Geometry check sheet. Reference: the model listing, model coordinates, mm. A direction names the side the tool comes from. Coordinates: 2 decimals unless noted, no trailing zeros. Loops run counter-clockwise (first coordinate to the right, second up) from the corner with the lowest first, then second, coordinate; pieces in that order, holes last. Notation, with made-up numbers: M 31,37 L 86,37 A13 cw 86,42 Z; hole C 44,42.5 d5. An arc over 180 degrees is marked long. Use CSV: the item, a comma, the result in double quotes.
```python
from build123d import *

# Parameters (mm, degrees)
F0_W     = 457.2
F0_H     = 139.7
F1_DEPTH = 19.05
F2_W     = 19.05
F2_H     = 12.7
F3_DEPTH = 139.701
F4_W     = 19.05
F4_H     = 12.7
F5_DEPTH = 139.701


with BuildPart() as f1:
    # F0 (on Front) → F1 (new body)
    with BuildSketch(Plane.XZ):
        with Locations((-228.6, 69.85)):
            Rectangle(F0_W, F0_H)
    extrude(amount=F1_DEPTH)

    # F2 (on face) → F3 (cut, through all)
    with BuildSketch(Plane.XY.offset(139.7)):
        with Locations((-9.525, -6.35)):
            Rectangle(F2_W, F2_H)
    extrude(amount=-F3_DEPTH, mode=Mode.SUBTRACT)

    # F4 (on face) → F5 (cut, through all)
    with BuildSketch(Plane.XY.offset(139.7)):
        with Locations((-447.675, -6.35)):
            Rectangle(F4_W, F4_H)
    extrude(amount=-F5_DEPTH, mode=Mode.SUBTRACT)


solid = f1.part
```
1. Set-up check for faces 1 (the flat face through (-232, 0, 71)), 2 (the flat face through (-19.05, -6, 71)), 3 (the flat face through (-438.15, -6, 71)): record each of +Z, -Z, +X, -X, +Y, -Y from which the full face is reachable in a straight line by a thin tool's end or side.
The answers:
face 1,"+Z, -Z, +X, -X, +Y"
face 2,"+Z, -Z, +X, +Y"
face 3,"+Z, -Z, -X, +Y"
2. Section check B-B, the plane y = -8.75. Record the cut outline in (x, z), plus the area to 3 significant figures.
The answers:
outline,"M -438.15,0 L -19.05,0 L -19.05,139.7 L -438.15,139.7 Z"
area,"58,500 mm^2"
3. Thickness scan on line 1 (X direction, y = -2.25, z = 72.5). Record the ranges inside material, lowest first. Write a range as [from, to].
The answers:
line 1,"[-438.15, -19.05]"
4. Gauge pin test, flat ends, axial feed: P1, Ø5, axis at y = -7.5, z = 93.5, coming from the -X side; P2, Ø21, axis at x = -451.5, z = 44, coming from the +Y side; P3, Ø6.5, axis at y = -7, z = 75, coming from the +X side. Record the tip position at first contact, or that the pin passes through.
The answers:
P1,"x = -438.15"
P2,"y = -12.7"
P3,"x = -19.05"
5. Section check A-A, the plane z = 33.5. Record the cut outline in (x, y), plus the area to 3 significant figures.
The answers:
outline,"M -457.2,-19.05 L 0,-19.05 L 0,-12.7 L -19.05,-12.7 L -19.05,0 L -438.15,0 L -438.15,-12.7 L -457.2,-12.7 Z"
area,"8,230 mm^2"
